Answer from the drawing. Dimensions are ordinates in mm from the lowest x, y and z of the part. Coordinates: 2 decimals unless noted, no trailing zeros. Loops run counter-clockwise (first coordinate to the right, second up) from the corner with the lowest first, then second, coordinate; pieces in that order, holes last.
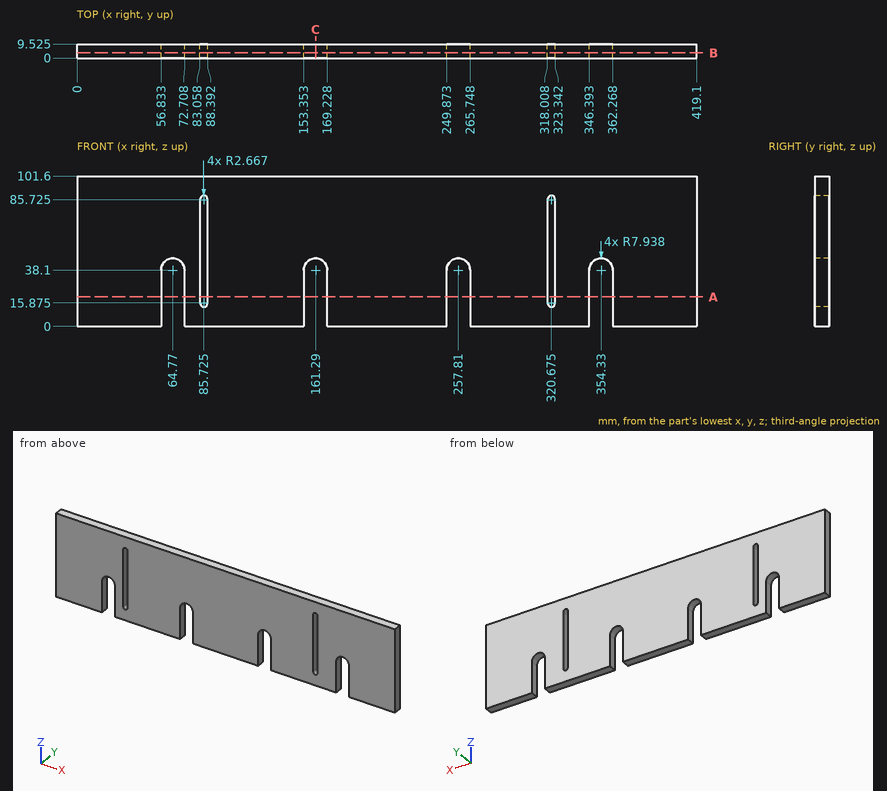
Item 1: Find the intervals of material crossed by line 1 along X through (y, z) = (7, 51.5); line 2 along Z through (x, y) = (355, 5.25); line 3 along Z through (x, y) = (71, 4.75) (1 decimal), in increasing order.
Numbers:
line 1: x = 0 to 83.06, 88.39 to 318.01, 323.34 to 419.1
line 2: z = 46.01 to 101.6
line 3: z = 43 to 101.6
Item 2: A cutting plane is placed at B-B on y = 3.5. Determine the outline of the cut face in (x, z) (1 decimal), then the cut area to 3 significant figures.
Numbers:
outline: (0, 0) - (56.8, 0) - (56.8, 38.1) arc R7.9 cw to (72.7, 38.1) - (72.7, 0) - (153.4, 0) - (153.4, 38.1) arc R7.9 cw to (169.2, 38.1) - (169.2, 0) - (249.9, 0) - (249.9, 38.1) arc R7.9 cw to (265.7, 38.1) - (265.7, 0) - (346.4, 0) - (346.4, 38.1) arc R7.9 cw to (362.3, 38.1) - (362.3, 0) - (419.1, 0) - (419.1, 101.6) - (0, 101.6) - close; hole (83.1, 15.9) arc R2.7 ccw to (88.4, 15.9) - (88.4, 85.7) arc R2.7 ccw to (83.1, 85.7) - close; hole (318, 15.9) arc R2.7 ccw to (323.3, 15.9) - (323.3, 85.7) arc R2.7 ccw to (318, 85.7) - close
area: 39,000 mm2
Item 3: A cutting plane is placed at C-C on x = 161.29. Determine the outline of the cut face in (y, z) (1 decimal).
Numbers:
outline: (0, 46) - (9.5, 46) - (9.5, 101.6) - (0, 101.6) - close
Item 4: A cutting plane is placed at A-A on z = 20. Determine the outline of the cut face in (x, y) (1 decimal).
Numbers:
outline: (0, 0) - (56.8, 0) - (56.8, 9.5) - (0, 9.5) - close; (72.7, 0) - (83.1, 0) - (83.1, 9.5) - (72.7, 9.5) - close; (88.4, 0) - (153.4, 0) - (153.4, 9.5) - (88.4, 9.5) - close; (169.2, 0) - (249.9, 0) - (249.9, 9.5) - (169.2, 9.5) - close; (265.7, 0) - (318, 0) - (318, 9.5) - (265.7, 9.5) - close; (323.3, 0) - (346.4, 0) - (346.4, 9.5) - (323.3, 9.5) - close; (362.3, 0) - (419.1, 0) - (419.1, 9.5) - (362.3, 9.5) - close
Item 5: Given pin 1 (1.5 mm diameter, centred on x = 59.5, y = 1.5, fed in from -Z) (1 decimal), flat-ended and moving along its own axis, determine where the tip first touches the part or whether it passes through.
Numbers:
pin 1: stops at z = 43.3
